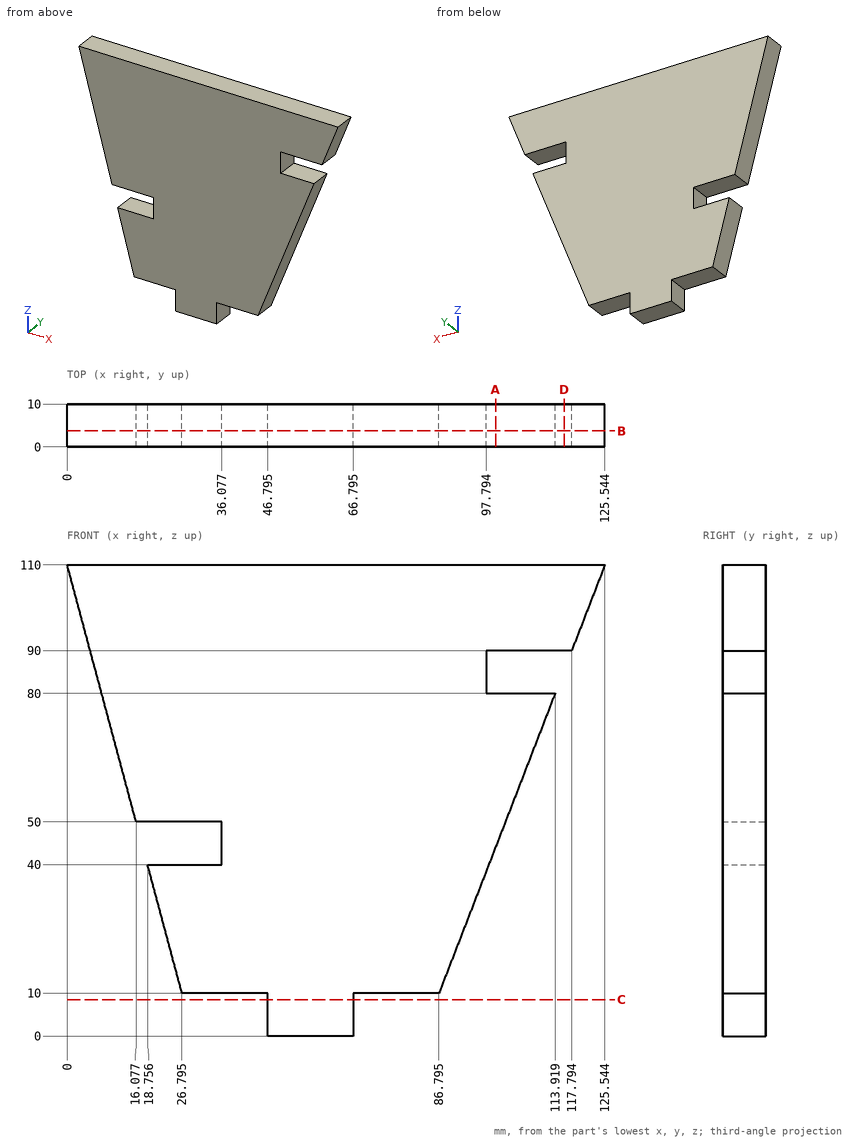
Verification items for this drawing (mm, ordinates from the low corner). Give positions to 0.01 mm unless a question says otherwise; leave off trailing zeros. Loops run counter-clockwise (first coordinate to the right, second up) from the corner with the lowest first, then second, coordinate; pieces in that order, holes last. Notation, with made-up numbers: M 51.5,88 L 73.5,88 A12 ccw 73.5,102 Z; hole C 82,57.25 d11. An arc over 180 degrees is marked long. Answer as a JSON object with one key per item and string values. Group by question number.
Q1. Cross-section at C-C on z = 8.5. Record the cut outline in (x, y) (1 decimal).
Q2. Cross-section at B-B on y = 3.75. Record the cut outline in (x, z) (1 decimal).
Q3. Cross-section at A-A on x = 100. Record the cut outline in (y, z), then the cut area to 3 significant figures.
Q4. Cross-section at D-D on x = 116. Record the cut outline in (y, z).
Q5. Material ranges on line 1 along Z through (x, y) = (83, 9.75); line 2 along Z through (x, y) = (18.5, 7.5); line 3 along X through (y, z) = (1.25, 80.5) (1 decimal), recorded low to high. Write a range as [from, to].
Q6. Go/stop test with flat-tipped pins: P1, Ø1.5, axis at y = 7.5, z = 78.5, coming from the +X side; P2, Ø1.5, axis at y = 5, z = 51.5, coming from the -X side; P3, Ø3, axis at y = 5, z = 3, coming from the +X side (1 decimal). Record where each tip stops, or that it passes through.
Evaluation:
{
 "1": {"outline": "M 46.8,0 L 66.8,0 L 66.8,10 L 46.8,10 Z"},
 "2": {"outline": "M 0,110 L 16.1,50 L 36.1,50 L 36.1,40 L 18.8,40 L 26.8,10 L 46.8,10 L 46.8,0 L 66.8,0 L 66.8,10 L 86.8,10 L 113.9,80 L 97.8,80 L 97.8,90 L 117.8,90 L 125.5,110 Z"},
 "3": {"outline": "M 0,44.08 L 10,44.08 L 10,80 L 0,80 Z; M 0,90 L 10,90 L 10,110 L 0,110 Z", "area": "559 mm2"},
 "4": {"outline": "M 0,90 L 10,90 L 10,110 L 0,110 Z"},
 "5": {"line 1": "z = [10, 110]", "line 2": "z = [50, 110]", "line 3": "x = [7.9, 97.8]"},
 "6": {"P1": "stops at x = 113.63", "P2": "stops at x = 15.47", "P3": "stops at x = 66.8"}
}
